Input: part model. Units: mm. Frame: model coordinates. Coordinates: 2 decimals unless noted, no trailing zeros. Order: outer loops, then holes, each group sorted by start corner. A loop starts at its lowest first (then second) coordinate and runs counter-clockwise, first axis right, second up. Notation, with made-up numbers: (-31, -22.75) -> (4, -22.75) arc R37 cw to (4, 14.25) -> close; hole circle Ø7 at (-14, 89.5). An arc over 180 degrees is marked (long way). Answer as CSV lines item,"result".
from build123d import *

# Parameters (mm, degrees)
SKETCH_1_W          = 164
SKETCH_1_H          = 164
EXTRUDE_1_DEPTH     = 1
FILLET_1_R          = 30
SKETCH_2_R          = 1.6
CUT_EXTRUDE_1_DEPTH = 2
SKETCH_3_R          = 1.6
CUT_EXTRUDE_2_DEPTH = 2
SKETCH_4_W          = 38
SKETCH_4_H          = 9
CUT_EXTRUDE_3_DEPTH = 2
SKETCH_5_W          = 1
SKETCH_5_H          = 9.5
CUT_EXTRUDE_4_DEPTH = 5
FILLET_3_R          = 1.5
SKETCH_6_W          = 29
SKETCH_6_H          = 11
EXTRUDE_2_DEPTH     = 1
FILLET_2_R          = 2
SKETCH_8_R          = 1.6
CUT_EXTRUDE_5_DEPTH = 2
SKETCH_10_R         = 1.599999996
SKETCH_10_R_2       = 1.600000004
SKETCH_10_R_3       = 1.35
CUT_EXTRUDE_6_DEPTH = 2
CUT_EXTRUDE_7_DEPTH = 2
FILLET_4_R          = 1.5


with BuildPart() as part:
    # 草图1 → 凸台-拉伸1 (new body)
    with BuildSketch(Plane.XY):
        with Locations((82, 82)):
            Rectangle(SKETCH_1_W, SKETCH_1_H)
    extrude(amount=EXTRUDE_1_DEPTH)

    # 圆角1
    fillet_1_edges = [part.edges().sort_by_distance(p)[0] for p in [
        (0, 164, 0.5),
        (0, 0, 0.5),
    ]]
    fillet(fillet_1_edges, radius=FILLET_1_R)

    # 草图2 → 切除-拉伸1 (cut, through all)
    with BuildSketch(Plane.XY.offset(1)):
        with Locations((5, 97)):
            Circle(SKETCH_2_R)
        with Locations((5, 67)):
            Circle(SKETCH_2_R)
        with BuildLine():
            Line((2, 77), (2, 87))
            ThreePointArc((2, 87), (5, 90), (8, 87))
            Line((8, 87), (8, 77))
            ThreePointArc((8, 77), (5, 74), (2, 77))
        make_face()
    extrude(amount=-CUT_EXTRUDE_1_DEPTH, mode=Mode.SUBTRACT)

    # 草图3 → 切除-拉伸2 (cut, through all)
    with BuildSketch(Plane.XY.offset(1)):
        with Locations((59, 5)):
            Circle(SKETCH_3_R)
        with Locations((89, 5)):
            Circle(SKETCH_3_R)
        with Locations((89, 159)):
            Circle(SKETCH_3_R)
        with Locations((59, 159)):
            Circle(SKETCH_3_R)
        with BuildLine():
            Line((79, 2), (69, 2))
            ThreePointArc((69, 2), (66, 5), (69, 8))
            Line((69, 8), (79, 8))
            ThreePointArc((79, 8), (82, 5), (79, 2))
        make_face()
        with BuildLine():
            Line((79, 162), (69, 162))
            ThreePointArc((69, 162), (66, 159), (69, 156))
            Line((69, 156), (79, 156))
            ThreePointArc((79, 156), (82, 159), (79, 162))
        make_face()
    extrude(amount=-CUT_EXTRUDE_2_DEPTH, mode=Mode.SUBTRACT)

    # 草图4 → 切除-拉伸3 (cut, through all)
    with BuildSketch(Plane.XY.offset(1)):
        with Locations((116, 159.5)):
            Rectangle(SKETCH_4_W, SKETCH_4_H)
        with Locations((116, 4.5)):
            Rectangle(SKETCH_4_W, SKETCH_4_H)
    extrude(amount=-CUT_EXTRUDE_3_DEPTH, mode=Mode.SUBTRACT)

    # 草图5 → 切除-拉伸4 (cut)
    with BuildSketch(Plane(origin=(164, 0, 0), x_dir=(0, 0, -1), z_dir=(1, 0, 0))):
        with Locations((-0.5, 67)):
            Rectangle(SKETCH_5_W, SKETCH_5_H)
        with Locations((-0.5, 97)):
            Rectangle(SKETCH_5_W, SKETCH_5_H)
    extrude(amount=-CUT_EXTRUDE_4_DEPTH, mode=Mode.SUBTRACT)

    # 圆角3
    fillet_3_edges = [part.edges().sort_by_distance(p)[0] for p in [
        (159, 62.25, 0.5),
        (159, 71.75, 0.5),
        (159, 101.75, 0.5),
        (159, 92.25, 0.5),
    ]]
    fillet(fillet_3_edges, radius=FILLET_3_R)

    # 草图6 → 凸台-拉伸2 (add)
    with BuildSketch(Plane.XY.offset(1)):
        with Locations((149.5, 169.5)):
            Rectangle(SKETCH_6_W, SKETCH_6_H)
        with Locations((149.5, -5.5)):
            Rectangle(SKETCH_6_W, SKETCH_6_H)
    extrude(amount=-EXTRUDE_2_DEPTH)

    # 圆角2
    fillet_2_edges = [part.edges().sort_by_distance(p)[0] for p in [
        (135, 155, 0.5),
        (97, 155, 0.5),
        (97, 164, 0.5),
        (97, 0, 0.5),
        (97, 9, 0.5),
        (135, 9, 0.5),
        (164, 71.75, 0.5),
        (164, 62.25, 0.5),
        (164, 92.25, 0.5),
        (164, 101.75, 0.5),
        (164, 175, 0.5),
        (135, 175, 0.5),
        (164, -11, 0.5),
        (135, -11, 0.5),
    ]]
    fillet(fillet_2_edges, radius=FILLET_2_R)

    # 草图8 → 切除-拉伸5 (cut, through all)
    with BuildSketch(Plane.XY.offset(1)):
        with Locations((156, 172)):
            Circle(SKETCH_8_R)
        with Locations((156, -8)):
            Circle(SKETCH_8_R)
    extrude(amount=-CUT_EXTRUDE_5_DEPTH, mode=Mode.SUBTRACT)

    # 草图10 → 切除-拉伸6 (cut, through all)
    with BuildSketch(Plane.XY.offset(1)):
        with Locations((71.449193661, 129.5)):
            Circle(SKETCH_10_R)
        with Locations((98.949193661, 129.5)):
            Circle(SKETCH_10_R)
        with Locations((126.449193661, 129.5)):
            Circle(SKETCH_10_R)
        with Locations((71.449193661, 82)):
            Circle(SKETCH_10_R)
        with Locations((126.449193661, 34.5)):
            Circle(SKETCH_10_R)
        with Locations((98.949193661, 34.5)):
            Circle(SKETCH_10_R)
        with Locations((71.449193661, 34.5)):
            Circle(SKETCH_10_R)
        with Locations((126.449193661, 82)):
            Circle(SKETCH_10_R_2)
        with Locations((28.449193661, 99.5)):
            Circle(SKETCH_10_R_3)
        with Locations((63.449193661, 99.5)):
            Circle(SKETCH_10_R_3)
        with Locations((63.449193661, 64.5)):
            Circle(SKETCH_10_R_3)
        with Locations((28.449193661, 64.5)):
            Circle(SKETCH_10_R_3)
        with Locations((146.449193661, 112)):
            Circle(SKETCH_10_R_3)
        with Locations((43.449193661, 112)):
            Circle(SKETCH_10_R_3)
        with Locations((63.449193661, 112)):
            Circle(SKETCH_10_R_3)
        with Locations((63.449193661, 52)):
            Circle(SKETCH_10_R_3)
        with Locations((43.449193661, 52)):
            Circle(SKETCH_10_R_3)
        with Locations((126.449193661, 112)):
            Circle(SKETCH_10_R_3)
        with Locations((146.449193661, 52)):
            Circle(SKETCH_10_R_3)
        with Locations((126.449193661, 52)):
            Circle(SKETCH_10_R_3)
    extrude(amount=-CUT_EXTRUDE_6_DEPTH, mode=Mode.SUBTRACT)

    # 草图12 → 切除-拉伸7 (cut, through all)
    with BuildSketch(Plane.XY.offset(1)):
        with BuildLine():
            Line((159, 94.5), (151.5, 94.5))
            Line((151.5, 94.5), (151.5, 69.5))
            Line((151.5, 69.5), (159, 69.5))
            Line((159, 69.5), (159, 70.25))
            ThreePointArc((159, 70.25), (159.439339828, 71.310660172), (160.5, 71.75))
            Line((160.5, 71.75), (162, 71.75))
            ThreePointArc((162, 71.75), (163.414213562, 72.335786438), (164, 73.75))
            Line((164, 73.75), (164, 90.25))
            ThreePointArc((164, 90.25), (163.414213562, 91.664213562), (162, 92.25))
            Line((162, 92.25), (160.5, 92.25))
            ThreePointArc((160.5, 92.25), (159.439339828, 92.689339828), (159, 93.75))
            Line((159, 93.75), (159, 94.5))
        make_face()
    extrude(amount=-CUT_EXTRUDE_7_DEPTH, mode=Mode.SUBTRACT)

    # 圆角4
    fillet_4_edges = [part.edges().sort_by_distance(p)[0] for p in [
        (159, 94.5, 0.5),
        (159, 69.5, 0.5),
        (151.5, 69.5, 0.5),
        (151.5, 94.5, 0.5),
    ]]
    fillet(fillet_4_edges, radius=FILLET_4_R)


solid = part.part
1. Contact query for flat-ended pins moving along their axis: pin 1 (0.5 mm diameter, centred on x = 73.5, z = 0.5, fed in from -Y); pin 2 (0.5 mm diameter, centred on x = 116, z = 0.5, fed in from -Y); pin 3 (0.5 mm diameter, centred on y = 162, z = 0.5, fed in from -X). Output: stop coordinate, or through.
Findings:
pin 1,"stops at y = 0"
pin 2,"stops at y = 9"
pin 3,"stops at x = 18.6"
2. Cut plane B-B (x = 33.5). Return the cut outline in (y, z), plus the area to 3 significant figures.
Findings:
outline,"(0, 0) -> (164, 0) -> (164, 1) -> (0, 1) -> close"
area,"164 mm2"
3. Ray query, line 1 along Y through (x, z) = (75, 0.5); line 2 along X through (y, z) = (82, 0.6); line 3 along Y through (x, z) = (59, 0.55). Return the intervals inside material, ascending.
Findings:
line 1,"y = 0 to 2, 8 to 156, 162 to 164"
line 2,"x = 0 to 2, 8 to 69.85, 73.05 to 124.85, 128.05 to 151.5"
line 3,"y = 0 to 3.4, 6.6 to 157.4, 160.6 to 164"
4. Cut plane A-A (z = 0.55). State how many separate pieces and enclosed holes the cut face has, plus the area to 3 significant figures.
Findings:
separate pieces,"1"
enclosed holes,"31"
area,"25,600 mm2"
